```python
from build123d import *

# Parameters (mm, degrees)
F1_DEPTH = 4.7625
F2_R     = 6.35
F2_R_2   = 3.96875
F2_R_3   = 4.7625
F3_DEPTH = 4.7635


with BuildPart() as f1:
    # F0 (on Front) → F1 (new body)
    with BuildSketch(Plane.XZ):
        Polygon((25.4, 0), (0, 0), (0, -50.8), (254, -50.8), (254, 0), (57.15, 47.625), (25.4, 47.625), align=None)
    extrude(amount=-F1_DEPTH)

    # F2 (on Front) → F3 (cut, through all)
    with BuildSketch(Plane.XZ):
        with Locations((228.6, -25.4)):
            Circle(F2_R)
        with Locations((74.6125, 30.1625)):
            Circle(F2_R_2)
        with Locations((50.8, 25.4)):
            Circle(F2_R_3)
    extrude(amount=-F3_DEPTH, mode=Mode.SUBTRACT)

    # F4: F1 across plane


with BuildPart() as f1_1:
    add(f1.part)
    add(f1.part.mirror(Plane.YZ))


solid = f1_1.part
```
CAD build for the part. Positions are in the model's coordinates, mm. Coordinates: 2 decimals unless noted, no trailing zeros. Loops run counter-clockwise (first coordinate to the right, second up) from the corner with the lowest first, then second, coordinate; pieces in that order, holes last. Notation, with made-up numbers: (11.5, 73.25) - (58.5, 73.25) arc R11 ccw to (58.5, 84.25) - close; hole circle Ø4 at (27, -14.5). An arc over 180 degrees is marked (long way). Return JSON: item names as keys, results as strings.
1. Band-saw the part on D-D (x = -10). Give the cut face in (y, z), and give its area (3 significant figures).
Result:
{"outline": "(0, -50.8) - (4.76, -50.8) - (4.76, 0) - (0, 0) - close", "area": "242 mm2"}
2. Drop a flat-ended pin along its axis: pin 1 (1.5 mm diameter, centred on x = -144, y = 3.5, fed in from +Z). Give the stop position or say it passes through.
Result:
{"pin 1": "stops at z = 26.79"}
3. Mould opens along X. For faces 1 (the flat face through (4, 4.762, -12)), 2 (the flat face through (156.95, 2.35, 23.48)), 3 (the cylindrical face through (-234.657, 2.348, -23.493)) say: released by +X, released by -X, zero draft, split by the parting line, or undercut.
Result:
{"face 1": "zero draft", "face 2": "released by +X", "face 3": "undercut"}
4. Probe L1, parallel to Z at x = 50.8, y = 1.75 (1 decimal); L2, parallel to Z at x = 223, y = 2.9; L3, parallel to Z at x = 179.5, y = 2.7. List the from-to ranges inside material, lowest first. Write a range as from..to.
Result:
{"L1": "z = -50.8..20.6, 30.2..47.6", "L2": "z = -50.8..-28.39, -22.41..7.5", "L3": "z = -50.8..18.02"}
5. Band-saw the part on C-C (z = 13). Give the cut face in (x, y).
Result:
{"outline": "(-200.27, 0) - (-25.4, 0) - (-25.4, 4.76) - (-200.27, 4.76) - close; (25.4, 0) - (200.27, 0) - (200.27, 4.76) - (25.4, 4.76) - close"}
6. Band-saw the part on B-B (y = 3.3). State how many separate pieces and enclosed holes the cut face has, and give its area (3 significant figures).
Result:
{"separate pieces": "1", "enclosed holes": "6", "area": "37,700 mm2"}
7. Band-saw the part on A-A (x = 50.8). Give the cut face in (y, z) (1 decimal), and give its area (3 significant figures).
Result:
{"outline": "(0, -50.8) - (4.8, -50.8) - (4.8, 20.6) - (0, 20.6) - close; (0, 30.2) - (4.8, 30.2) - (4.8, 47.6) - (0, 47.6) - close", "area": "423 mm2"}
